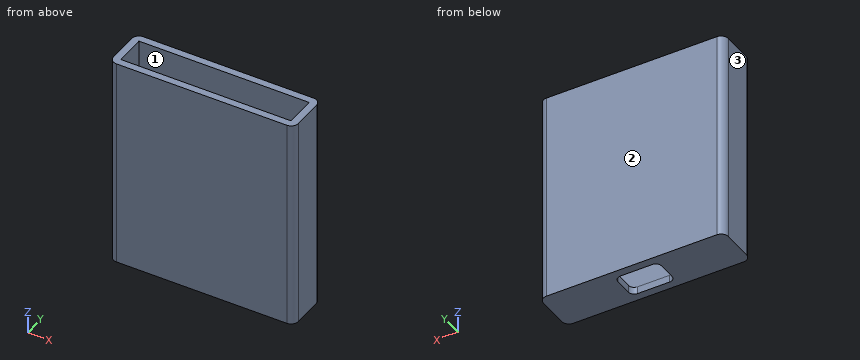
```python
from build123d import *

# Parameters (mm, degrees)
SKETCH1_W           = 32.385
SKETCH1_H           = 7.874
SKETCH1_W_2         = 29.845
SKETCH1_H_2         = 5.334
BOSS_EXTRUDE1_DEPTH = 37.338
FILLET1_R           = 1.27
SKETCH2_W           = 29.845
SKETCH2_H           = 5.334
BOSS_EXTRUDE2_DEPTH = 1.27


with BuildPart() as part:
    # Sketch1 → Boss-Extrude1 (new body)
    with BuildSketch(Plane.XY):
        Rectangle(SKETCH1_W, SKETCH1_H)
        Rectangle(SKETCH1_W_2, SKETCH1_H_2, mode=Mode.SUBTRACT)
    extrude(amount=-BOSS_EXTRUDE1_DEPTH)

    # Fillet1
    fillet1_edges = [part.edges().sort_by_distance(p)[0] for p in [
        (16.1925, -3.937, -18.669),
        (-16.1925, -3.937, -18.669),
        (-16.1925, 3.937, -18.669),
        (16.1925, 3.937, -18.669),
    ]]
    fillet(fillet1_edges, radius=FILLET1_R)

    # Sketch2 → Boss-Extrude2 (add)
    with BuildSketch(Plane(origin=(0, 0, -37.338), x_dir=(-1, 0, 0), z_dir=(0, 0, -1))):
        Rectangle(SKETCH2_W, SKETCH2_H)
        with BuildLine():
            Line((-2.794, 2.54), (2.794, 2.54))
            ThreePointArc((2.794, 2.54), (3.51242049, 2.24242049), (3.81, 1.524))
            Line((3.81, 1.524), (3.81, -1.524))
            ThreePointArc((3.81, -1.524), (3.51242049, -2.24242049), (2.794, -2.54))
            Line((2.794, -2.54), (-2.794, -2.54))
            ThreePointArc((-2.794, -2.54), (-3.51242049, -2.24242049), (-3.81, -1.524))
            Line((-3.81, -1.524), (-3.81, 1.524))
            ThreePointArc((-3.81, 1.524), (-3.51242049, 2.24242049), (-2.794, 2.54))
        make_face(mode=Mode.SUBTRACT)
    extrude(amount=-BOSS_EXTRUDE2_DEPTH)


solid = part.part
```
Geometry check sheet. Reference: the model listing, model coordinates, mm. Face numbers are marked on the shaded views. Round coordinates to 2 decimals unless told otherwise and drop trailing zeros. Loops run counter-clockwise (first coordinate to the right, second up) from the corner with the lowest first, then second, coordinate; pieces in that order, holes last. Notation, with made-up numbers: (-16.75, 52.25) -> (38.25, 52.25) arc R23 ccw to (38.25, 89.25) -> close; hole circle Ø5 at (-27, 15). An arc over 180 degrees is marked (long way). Use a Markdown table: item, result.
(1) Sectioned sample at D-D (y = 2). Enter the section's corners in (x, z).
Calculated:
| item | result |
|---|---|
| outline | (-16.19, -37.34) -> (-3.69, -37.34) -> (-3.69, -36.07) -> (-14.92, -36.07) -> (-14.92, 0) -> (-16.19, 0) -> close; (3.69, -37.34) -> (16.19, -37.34) -> (16.19, 0) -> (14.92, 0) -> (14.92, -36.07) -> (3.69, -36.07) -> close |
(2) Sectioned sample at C-C (x = 6.5). Enter the section's corners in (y, z), then the cut area to 3 significant figures.
Calculated:
| item | result |
|---|---|
| outline | (-3.94, -37.34) -> (3.94, -37.34) -> (3.94, 0) -> (2.67, 0) -> (2.67, -36.07) -> (-2.67, -36.07) -> (-2.67, 0) -> (-3.94, 0) -> close |
| area | 102 mm² |
(3) Sectioned sample at B-B (z = -20.5). Enter the section's corners in (x, y).
Calculated:
| item | result |
|---|---|
| outline | (-16.19, -2.67) arc R1.27 ccw to (-14.92, -3.94) -> (14.92, -3.94) arc R1.27 ccw to (16.19, -2.67) -> (16.19, 2.67) arc R1.27 ccw to (14.92, 3.94) -> (-14.92, 3.94) arc R1.27 ccw to (-16.19, 2.67) -> close; hole (-14.92, -2.67) -> (14.92, -2.67) -> (14.92, 2.67) -> (-14.92, 2.67) -> close |
(4) Sectioned sample at A-A (y = -1). Enter the section's corners in (x, z).
Calculated:
| item | result |
|---|---|
| outline | (-16.19, -37.34) -> (-3.81, -37.34) -> (-3.81, -36.07) -> (-14.92, -36.07) -> (-14.92, 0) -> (-16.19, 0) -> close; (3.81, -37.34) -> (16.19, -37.34) -> (16.19, 0) -> (14.92, 0) -> (14.92, -36.07) -> (3.81, -36.07) -> close |
(5) Mould release check, pull along Y, two halves, no side actions. Record for the marked faces 1, 2 and 3: released by +Y, released by -Y, zero draft, split by the parting line, or undercut.
Calculated:
| item | result |
|---|---|
| face 1 | undercut |
| face 2 | released by +Y |
| face 3 | zero draft |
(6) Scan lines: probe 1 along Y at (x, z) = (3, -22); probe 2 along X at (y, z) = (1.5, -17.5); probe 3 along Z at (x, y) = (-4.5, 1.5). Record each from-to range of solid material in increasing order.
Calculated:
| item | result |
|---|---|
| probe 1 | -3.94 to -2.67, 2.67 to 3.94 |
| probe 2 | -16.19 to -14.92, 14.92 to 16.19 |
| probe 3 | -37.34 to -36.07 |
(7) Go/stop test with a flat-tipped pin: P1, Ø4.5, axis at x = 6, y = 1, coming from the +Z side. Record where the tip stops, or that it passes through.
Calculated:
| item | result |
|---|---|
| P1 | z = 0 |
